Can you work these out from the drawing? Everything is in mm from the part's minimum corner. Coordinates: 2 decimals unless noted, no trailing zeros. Write each loop counter-clockwise with the first axis right and the second up, starting at its lowest first coordinate (ties: lowest second). Pieces come first, ordered by that corner, then holes. Notation, with made-up numbers: (-28.75, 80.25) -> (-15.75, 80.25) arc R20 cw to (-15.75, 115.25) -> close; hole circle Ø6 at (32.5, 55). An arc over 180 degrees is marked (long way). Use a Markdown table: item, result. Add a question column.
Item 1: Imagine slicing it at A-A, the plane y = 51.5. Write out the boundary of the cut face in (x, z).
Item 2: Will these pins go through, and if not, where does the flat tip stop? pin 1 Ø0.9 at (y, z) = (13, 1) entering from +X; pin 2 Ø0.9 at (y, z) = (54.5, 2) entering from -X.
Item 3: Imagine slicing it at B-B, the plane x = 22. Write out the boundary of the cut face in (y, z).
Item 4: If I drill on line 1 along X through (y, z) = (52, 1.3); line 2 along Y through (x, z) = (22.5, 1.55), over which ranges is the centre line in solid material (lowest first)? Write a range as from..to.
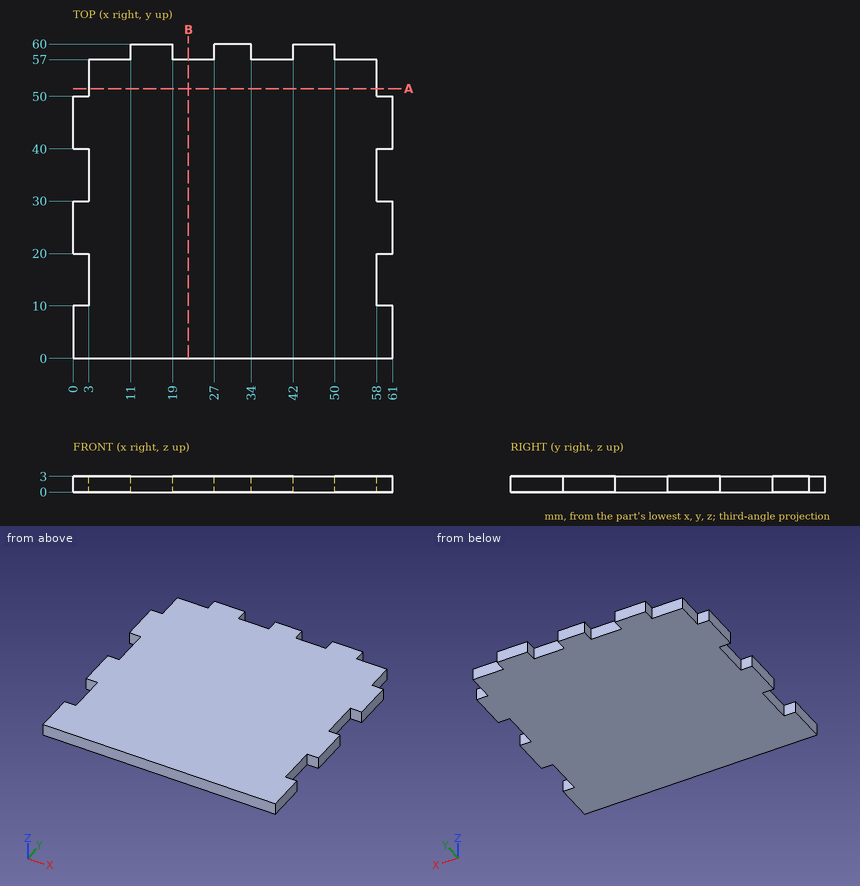
Ans:
| question | item | result |
|---|---|---|
| 1 | outline | (3, 0) -> (58, 0) -> (58, 3) -> (3, 3) -> close |
| 2 | pin 1 | stops at x = 58 |
| 2 | pin 2 | stops at x = 3 |
| 3 | outline | (0, 0) -> (57, 0) -> (57, 3) -> (0, 3) -> close |
| 4 | line 1 | x = 3..58 |
| 4 | line 2 | y = 0..57 |
